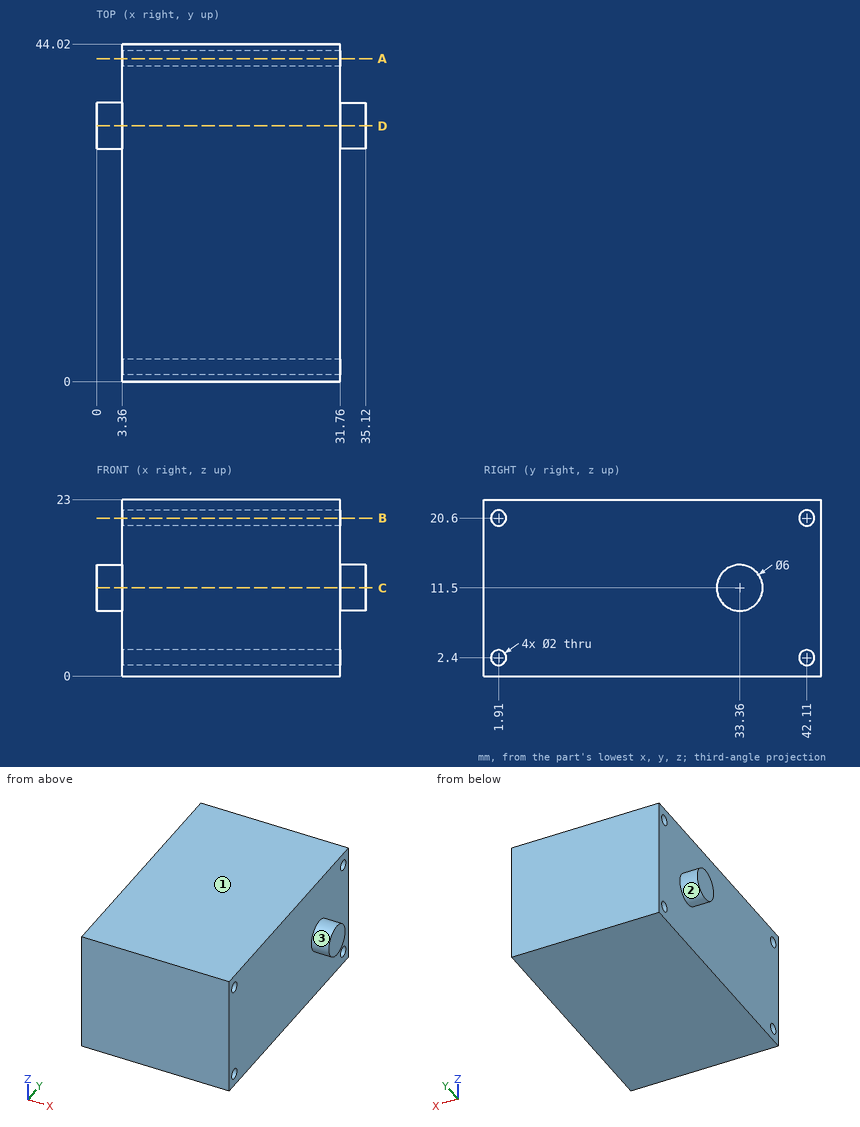
The figure shows three views and two pictorial views of one solid part (mm, origin at its lowest corner). Answer the questions. A direction names the side the tool comes from. Coordinates: 2 decimals unless noted, no trailing zeros. Write each loop counter-clockwise with the first axis right and the second up, starting at its lowest first coordinate (ties: lowest second). Pieces come first, ordered by that corner, then holes. Notation, with made-up numbers: M -11.5,19.25 L 18.5,19.25 A18 cw 18.5,47.25 Z; hole C 6.25,27 d6. An arc over 180 degrees is marked long. Answer as CSV lines item,"result". Start each with the question number.
Item 1: A tool of negligible diameter and unlimited length cuts with its end or side. For the marked faces 1, 2 and 3, from which of +Z, -Z, +X, -X, +Y, -Y can it reach the whole face along a straight path? Write none if from no direction.
Item 2: Section D-D on y = 33.36 is taken. Write down the section's boundary in (x, z), and give its area (3 significant figures).
Item 3: Flat-ended cylindrical pins translate along their axes: P1, Ø8, axis at y = 18, z = 14.5, coming from the +X side; P2, Ø3, axis at y = 30, z = 12, coming from the -X side; P3, Ø7, axis at y = 17.5, z = 15.5, coming from the -X side. Find the tip coordinate at first contact, or state that the pin passes through.
Item 4: Section C-C on z = 11.5 is taken. Write down the section's boundary in (x, y).
Item 5: Consider L1, parallel to Y at x = 17, z = 20.6; L2, parallel to Z at x = 11.25, y = 42.11; L3, parallel to Z at x = 20, y = 1. Determine where each line is inside the solid, lowest interval first.
Item 6: Section A-A on y = 42.11 is taken. Write down the section's boundary in (x, z).
Item 7: Section B-B on z = 20.6 is taken. Write down the section's boundary in (x, y).
Checks:
1,face 1,"+Z, +X, -X, +Y, -Y"
1,face 2,"-X"
1,face 3,"+X"
2,outline,"M 0,8.5 L 3.36,8.5 L 3.36,0 L 31.76,0 L 31.76,8.5 L 35.12,8.5 L 35.12,14.5 L 31.76,14.5 L 31.76,23 L 3.36,23 L 3.36,14.5 L 0,14.5 Z"
2,area,"694 mm²"
3,P1,"stops at x = 31.76"
3,P2,"stops at x = 0"
3,P3,"stops at x = 3.36"
4,outline,"M 0,30.36 L 3.36,30.36 L 3.36,0 L 31.76,0 L 31.76,30.36 L 35.12,30.36 L 35.12,36.36 L 31.76,36.36 L 31.76,44.02 L 3.36,44.02 L 3.36,36.36 L 0,36.36 Z"
5,L1,"y = 0 to 0.91, 2.91 to 41.11, 43.11 to 44.02"
5,L2,"z = 0 to 1.4, 3.4 to 19.6, 21.6 to 23"
5,L3,"z = 0 to 1.99, 2.81 to 20.19, 21.01 to 23"
6,outline,"M 3.36,0 L 31.76,0 L 31.76,1.4 L 3.36,1.4 Z; M 3.36,3.4 L 31.76,3.4 L 31.76,19.6 L 3.36,19.6 Z; M 3.36,21.6 L 31.76,21.6 L 31.76,23 L 3.36,23 Z"
7,outline,"M 3.36,0 L 31.76,0 L 31.76,0.91 L 3.36,0.91 Z; M 3.36,2.91 L 31.76,2.91 L 31.76,41.11 L 3.36,41.11 Z; M 3.36,43.11 L 31.76,43.11 L 31.76,44.02 L 3.36,44.02 Z"
